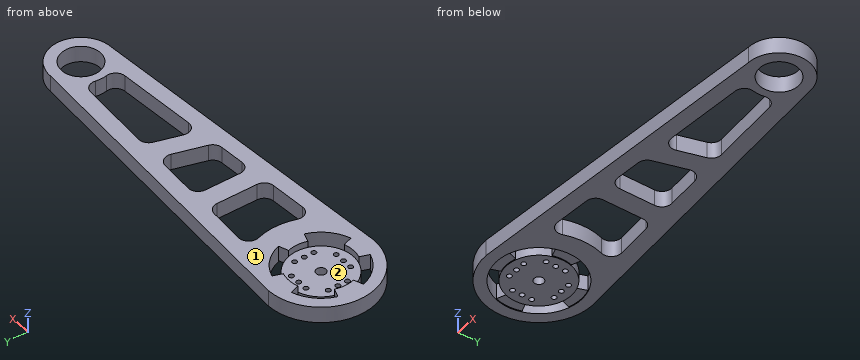
```python
from build123d import *
from build123d.topology import SkipClean

# Parameters (mm, degrees)
SKETCH_1_R          = 6
EXTRUDE_1_DEPTH     = 5
SKETCH_2_R          = 1.5
SKETCH_2_R_2        = 0.75
CUT_EXTRUDE_3_DEPTH = 86.605569128
CUT_EXTRUDE_6_DEPTH = 0.3
CUT_EXTRUDE_8_DEPTH = 86.605569128
CUT_EXTRUDE_START   = -2
SKETCH_9_R          = 10
CUT_EXTRUDE_9_DEPTH = 2


with BuildPart() as part:
    # 草图1 → 凸台-拉伸1 (new body)
    with BuildSketch(Plane.XY):
        with BuildLine():
            Line((-67.351436873, 16.5), (32.648563127, 9.5))
            ThreePointArc((32.648563127, 9.5), (42.148563127, 0), (32.648563127, -9.5))
            Line((32.648563127, -9.5), (-67.351436873, -16.5))
            ThreePointArc((-67.351436873, -16.5), (-83.851436873, 0), (-67.351436873, 16.5))
        make_face()
        with Locations((32.648563127, 0)):
            Circle(SKETCH_1_R, mode=Mode.SUBTRACT)
    extrude(amount=EXTRUDE_1_DEPTH)

    # 草图2 → 切除-拉伸3 (cut, through all)
    with BuildSketch(Plane(origin=(0, 0, 0), x_dir=(-1, 0, 0), z_dir=(0, 0, -1))):
        with Locations((67.351436873, 0)):
            Circle(SKETCH_2_R)
        with Locations((60.351436873, 0)):
            Circle(SKETCH_2_R_2)
        with Locations((60.351436873, 3)):
            Circle(SKETCH_2_R_2)
        with Locations((60.351436873, -3)):
            Circle(SKETCH_2_R_2)
        with Locations((70.351436873, 7)):
            Circle(SKETCH_2_R_2)
        with Locations((67.351436873, 7)):
            Circle(SKETCH_2_R_2)
        with Locations((64.351436873, 7)):
            Circle(SKETCH_2_R_2)
        with Locations((74.351436873, -3)):
            Circle(SKETCH_2_R_2)
        with Locations((74.351436873, 0)):
            Circle(SKETCH_2_R_2)
        with Locations((74.351436873, 3)):
            Circle(SKETCH_2_R_2)
        with Locations((64.351436873, -7)):
            Circle(SKETCH_2_R_2)
        with Locations((67.351436873, -7)):
            Circle(SKETCH_2_R_2)
        with Locations((70.351436873, -7)):
            Circle(SKETCH_2_R_2)
        with BuildLine():
            Line((70.351436873, 9.539392014), (71.378274732, 12.360605845))
            ThreePointArc((71.378274732, 12.360605845), (76.543825029, 9.192388155), (79.712042718, 4.026837859))
            Line((79.712042718, 4.026837859), (76.890828887, 3))
            ThreePointArc((76.890828887, 3), (74.422504685, 7.071067812), (70.351436873, 9.539392014))
        make_face()
        with BuildLine():
            Line((64.351436873, 9.539392014), (63.324599014, 12.360605845))
            ThreePointArc((63.324599014, 12.360605845), (58.159048718, 9.192388155), (54.990831028, 4.026837859))
            Line((54.990831028, 4.026837859), (57.812044859, 3))
            ThreePointArc((57.812044859, 3), (60.280369061, 7.071067812), (64.351436873, 9.539392014))
        make_face()
        with BuildLine():
            Line((76.890828887, -3), (79.712042718, -4.026837859))
            ThreePointArc((79.712042718, -4.026837859), (76.543825029, -9.192388155), (71.378274732, -12.360605845))
            Line((71.378274732, -12.360605845), (70.351436873, -9.539392014))
            ThreePointArc((70.351436873, -9.539392014), (74.422504685, -7.071067812), (76.890828887, -3))
        make_face()
        with BuildLine():
            Line((64.351436873, -9.539392014), (63.324599014, -12.360605845))
            ThreePointArc((63.324599014, -12.360605845), (58.159048718, -9.192388155), (54.990831028, -4.026837859))
            Line((54.990831028, -4.026837859), (57.812044859, -3))
            ThreePointArc((57.812044859, -3), (60.280369061, -7.071067812), (64.351436873, -9.539392014))
        make_face()
    extrude(amount=-CUT_EXTRUDE_3_DEPTH, mode=Mode.SUBTRACT)

    # 草图5 → 切除-拉伸6 (cut)
    with SkipClean():  # the faces are left unmerged after this step: merging them gives an invalid solid
        with BuildSketch(Plane(origin=(0, 0, 0), x_dir=(-1, 0, 0), z_dir=(0, 0, -1))):
            with BuildLine():
                Line((70.351436873, -9.539392014), (71.378274732, -12.360605845))
                ThreePointArc((71.378274732, -12.360605845), (67.351436873, -13), (63.324599014, -12.360605845))
                Line((63.324599014, -12.360605845), (64.351436873, -9.539392014))
                ThreePointArc((64.351436873, -9.539392014), (67.351436873, -10), (70.351436873, -9.539392014))
            make_face()
            with BuildLine():
                Line((57.812044859, -3), (54.990831028, -4.026837859))
                ThreePointArc((54.990831028, -4.026837859), (54.351436873, 0), (54.990831028, 4.026837859))
                Line((54.990831028, 4.026837859), (57.812044859, 3))
                ThreePointArc((57.812044859, 3), (57.351436873, 0), (57.812044859, -3))
            make_face()
            with BuildLine():
                Line((79.712042718, -4.026837859), (76.890828887, -3))
                ThreePointArc((76.890828887, -3), (77.351436873, 0), (76.890828887, 3))
                Line((76.890828887, 3), (79.712042718, 4.026837859))
                ThreePointArc((79.712042718, 4.026837859), (80.351436873, 0), (79.712042718, -4.026837859))
            make_face()
            with BuildLine():
                Line((71.378274732, 12.360605845), (70.351436873, 9.539392014))
                ThreePointArc((70.351436873, 9.539392014), (67.351436873, 10), (64.351436873, 9.539392014))
                Line((64.351436873, 9.539392014), (63.324599014, 12.360605845))
                ThreePointArc((63.324599014, 12.360605845), (67.351436873, 13), (71.378274732, 12.360605845))
            make_face()
        extrude(amount=-CUT_EXTRUDE_6_DEPTH, mode=Mode.SUBTRACT)

    # 草图7 → 切除-拉伸8 (cut, through all)
    with SkipClean():  # the faces are left unmerged after this step: merging them gives an invalid solid
        with BuildSketch(Plane.XY.offset(5)):
            with BuildLine():
                Line((-32.351436873, 6.240423951), (-32.351436873, -6.279908436))
                ThreePointArc((-32.351436873, -6.279908436), (-33.159771035, -8.328469115), (-35.149170775, -9.273082074))
                Line((-35.149170775, -9.273082074), (-46.303856397, -10.026868861))
                ThreePointArc((-46.303856397, -10.026868861), (-48.882666549, -8.864552498), (-49.348665365, -6.074554966))
                ThreePointArc((-49.348665365, -6.074554966), (-48.351437761, -0.005807318), (-49.344955374, 6.063548799))
                ThreePointArc((-49.344955374, 6.063548799), (-48.875599725, 8.855399851), (-46.292339334, 10.013628142))
                Line((-46.292339334, 10.013628142), (-35.14194949, 9.233100853))
                ThreePointArc((-35.14194949, 9.233100853), (-33.157301263, 8.286339132), (-32.351436873, 6.240423951))
            make_face()
            with BuildLine():
                Line((-23.14194949, 8.393100853), (-12.658599808, 7.659266375))
                ThreePointArc((-12.658599808, 7.659266375), (-10.408556973, 6.384352876), (-9.986244931, 3.832931757))
                Line((-9.986244931, 3.832931757), (-12.767703456, -5.782195127))
                ThreePointArc((-12.767703456, -5.782195127), (-13.767045159, -7.284386647), (-15.447279617, -7.941711049))
                Line((-15.447279617, -7.941711049), (-23.149170775, -8.462172493))
                ThreePointArc((-23.149170775, -8.462172493), (-25.399997551, -7.660664694), (-26.351436873, -5.468998855))
                Line((-26.351436873, -5.468998855), (-26.351436873, 5.400423951))
                ThreePointArc((-26.351436873, 5.400423951), (-25.397352054, 7.594559561), (-23.14194949, 8.393100853))
            make_face()
            with BuildLine():
                Line((-3.505857343, 4.643162142), (-5.790312558, -3.25389135))
                ThreePointArc((-5.790312558, -3.25389135), (-5.244319535, -5.970049623), (-2.7062042, -7.080722705))
                Line((-2.7062042, -7.080722705), (21.637024401, -5.435709596))
                ThreePointArc((21.637024401, -5.435709596), (23.82451027, -4.256119574), (24.371955288, -1.831901968))
                ThreePointArc((24.371955288, -1.831901968), (24.183794233, -0.066811207), (24.345729084, 1.700878551))
                ThreePointArc((24.345729084, 1.700878551), (23.778220575, 4.09624397), (21.609277414, 5.26051497))
                Line((21.609277414, 5.26051497), (-0.414527699, 6.802181327))
                ThreePointArc((-0.414527699, 6.802181327), (-2.341778485, 6.269034644), (-3.505857343, 4.643162142))
            make_face()
        extrude(amount=-CUT_EXTRUDE_8_DEPTH, mode=Mode.SUBTRACT)

    # 草图9 → 切除-拉伸9 (cut)
    with SkipClean():  # the faces are left unmerged after this step: merging them gives an invalid solid
        with BuildSketch(Plane.XY.offset(5).offset(CUT_EXTRUDE_START)):
            with Locations(Location((-67.351436873, 0, 0), (0, 0, 180))):
                Circle(SKETCH_9_R)
        extrude(amount=CUT_EXTRUDE_9_DEPTH, mode=Mode.SUBTRACT)


solid = part.part
```
Can you work these out from the model? Positions are in its coordinate system, mm. Face numbers are marked on the shaded views. Coordinates: 2 decimals unless noted, no trailing zeros. Loops run counter-clockwise (first coordinate to the right, second up) from the corner with the lowest first, then second, coordinate; pieces in that order, holes last. Notation, with made-up numbers: (75.5, 84.25) -> (100.5, 84.25) arc R22 cw to (100.5, 96.25) -> close; hole circle Ø9 at (-39.75, 50.5). An arc over 180 degrees is marked (long way). Put each result on its own line as item: value. Start each with the question number.
Q1. I'm going to push flat-ended pins straight in: P1, Ø1.7, axis at x = -64.35, y = 7, coming from the +Z side; P2, Ø1.5, axis at y = -1.5, z = 1.5, coming from the +X side; P3, Ø2, axis at x = -59.5, z = 1.5, coming from the -Y side. Where does each tip first touch, or does it pass through?
Q2. Thinking about a two-plate mould opening in X: for the marked faces 1 and 2, which applies, pulls with the +X half, pulls with the -X half, needs draft (parallel to the pull), parting line crosses it, or undercut?
Q3. If I drill on line 1 (Y direction, x = -60.5, z = 0.8); line 2 (X direction, y = 5, z = 4.7); line 3 (Y direction, x = -56, z = 3.95), over which ranges is the centre line in solid material (lowest first)? Write a range as [from, to].
Q4. I want a section at A-A (x = 29). Write out the boundary of the cut face in (y, z).
Taken from the geometry:
1. P1: stops at z = 3
1. P2: stops at x = 42.12
1. P3: stops at y = -16.02
2. face 1: needs draft
2. face 2: undercut
3. line 1: y = [-16.02, -11.05], [-7.28, -3.74], [-2.26, -0.74], [0.74, 2.26], [3.74, 7.28], [11.05, 16.02]
3. line 2: x = [-83.08, -79.35], [-55.35, -49.02], [-32.35, -26.35], [-9.89, -3.38], [22.64, 29.33], [35.97, 40.73]
3. line 3: y = [-15.71, -6.34], [-3.66, 3.66], [6.34, 15.71]
4. outline: (-9.76, 0) -> (-4.76, 0) -> (-4.76, 5) -> (-9.76, 5) -> close; (4.76, 0) -> (9.76, 0) -> (9.76, 5) -> (4.76, 5) -> close
